Geometry check sheet. Reference: the model listing, model coordinates, mm. A direction names the side the tool comes from. Round coordinates to 2 decimals unless told otherwise and drop trailing zeros. Order: outer loops, then holes, each group sorted by start corner. A loop starts at its lowest first (then second) coordinate and runs counter-clockwise, first axis right, second up.
Autodesk Inventor part; units mm, degrees
ref_plane "YZ Plane" through (0, 0, 0) normal (1, 0, 0) x (0, 1, 0)
ref_plane "XZ Plane" through (0, 0, 0) normal (0, 1, 0) x (-1, 0, 0)
ref_plane "XY Plane" through (0, 0, 0) normal (0, 0, 1) x (1, 0, 0)
sketch "スケッチ1" plane through (0, 0, 0) normal (0, 0, 1) x (1, 0, 0)
  circle A0 centre (0, 0) radius 2
  dimension "d0" = 4
extrude "押し出し1" add sketch "スケッチ1" along normal blind 12
thread "ねじ1"
sketch "スケッチ2" plane through (0, 0, 12) normal (0, 0, 1) x (1, 0, 0)
  circle A0 centre (0, 0) radius 4
  dimension "d5" = 8
extrude "押し出し2" add sketch "スケッチ2" along normal blind 1.5
sketch "スケッチ3" plane through (0, 0, 13.5) normal (0, 0, 1) x (1, 0, 0)
  line L0 (0, 1.1547) -> (1, 0.5774)
  line L1 (1, 0.5774) -> (1, -0.5774)
  line L2 (1, -0.5774) -> (0, -1.1547)
  line L3 (0, -1.1547) -> (-1, -0.5774)
  line L4 (-1, -0.5774) -> (-1, 0.5774)
  line L5 (-1, 0.5774) -> (0, 1.1547)
  point P0 (0, 0)
  point P1 (0, 0)
  dimension "d8" = 2
extrude "押し出し3" cut sketch "スケッチ3" against normal blind 2.5
properties part number "M4極低頭ネジ　12" material "鋼、高強度、低合金"
(1) Sectioned sample at C-C, the plane x = -2.25. Record the cut outline in (y, z), and give its area (3 significant figures).
Returned:
outline: (-3.31, 12) - (3.31, 12) - (3.31, 13.5) - (-3.31, 13.5) - close
area: 9.92 mm2
(2) Draft check along X on faces 4 (the flat face through (1, -1, 13.5)), 5 (the flat face through (0.49, 0.87, 12.27)), 6 (the cylindrical face through (0, 2, 6)). Enter one of: released by +X, released by -X, zero draft, split by the parting line, or undercut.
Returned:
face 4: zero draft
face 5: undercut
face 6: split by the parting line
(3) Sectioned sample at A-A, the plane y = 0. Record the cut outline in (x, z), and give its area (3 significant figures).
Returned:
outline: (-4, 12) - (-2, 12) - (-2, 0) - (2, 0) - (2, 12) - (4, 12) - (4, 13.5) - (1, 13.5) - (1, 11) - (-1, 11) - (-1, 13.5) - (-4, 13.5) - close
area: 55.0 mm2
(4) Material ranges on line 1 (Y direction, x = 0, z = 9.25); line 2 (Z direction, x = 3.25, y = 2); line 3 (Z direction, x = 0.25, y = 0.5), recorded low to high.
Returned:
line 1: y = -2 to 2
line 2: z = 12 to 13.5
line 3: z = 0 to 11
(5) Depth check by flat-ended pin: P1, Ø1, axis at x = 2.5, y = -1.5, coming from the -Z side; P2, Ø1.5, axis at y = 0.5, z = 9, coming from the -X side; P3, Ø0.6, axis at y = 0, z = 11.5, coming from the +X side; P4, Ø1.6, axis at x = 0, y = -0.5, coming from the +Z side. Enter the tip coordinate at first touch or a pass-through.
Returned:
P1: stops at z = 12
P2: stops at x = -2
P3: stops at x = 2
P4: stops at z = 13.5
(6) Sectioned sample at B-B, the plane z = 11.5. Record the cut outline in (x, y).
Returned:
outline: circle Ø4 at (0, 0); hole (-1, -0.58) - (0, -1.15) - (1, -0.58) - (1, 0.58) - (0, 1.15) - (-1, 0.58) - close
(7) Sectioned sample at D-D, the plane y = 2.5. Record the cut outline in (x, z), and give its area (3 significant figures).
Returned:
outline: (-3.12, 12) - (3.12, 12) - (3.12, 13.5) - (-3.12, 13.5) - close
area: 9.37 mm2
(8) Set-up check for faces 1 (the flat face through (0, 0, 0)), 2 (the flat face through (-2, -1, 12)), 3 (the flat face through (-1, 0, 12)): record each of +Z, -Z, +X, -X, +Y, -Y from which the full face is reachable in a straight line by a thin tool's end or side.
Returned:
face 1: -Z, +X, -X, +Y, -Y
face 2: -Z
face 3: +Z
